Geometry check sheet. Reference: the model listing, model coordinates, mm. Round coordinates to 2 decimals unless told otherwise and drop trailing zeros. Write each loop counter-clockwise with the first axis right and the second up, starting at its lowest first coordinate (ties: lowest second). Pieces come first, ordered by that corner, then holes. Notation, with made-up numbers: M 14,87.5 L 20,87.5 A18 cw 20,101.5 Z; hole C 14.5,61 d9. An arc over 180 degrees is marked long. One line per item, written item: value. Start each with the question number.
1. Depth check by flat-ended pin: P1, Ø5, axis at y = -12, z = 37.5, coming from the +X side; P2, Ø6, axis at y = -19.5, z = 45.5, coming from the +X side; P3, Ø10, axis at y = -15, z = 27, coming from the -X side. Enter the tip coordinate at first touch or a pass-through.
2. Release check for a two-part mould opening along Z. For faces 1 (the flat face through (207, -23, 68)), 2 (the cylindrical face through (282.717, -11.339, -26.81)), 3 (the cylindrical face through (279.922, -11.099, -25.652)) record: pulls with the +Z half, pulls with the -Z half, needs draft (parallel to the pull), parting line crosses it, or undercut.
3. Section check A-A (z = 0). Record the boundary of the cut face in (x, y), and give its area (3 significant figures).
4. Scan lines: probe 1 along X at (y, z) = (-8.5, 18.5); probe 2 along Z at (x, y) = (224.5, -13.5); probe 3 along Z at (x, y) = (197.5, -2.5). Record each from-to range of solid material in increasing order. Write a range as [from, to].
5. Section check B-B (y = -13.5). Record the boundary of the cut face in (x, z) (3 decimals).
from build123d import *

# Parameters (mm, degrees)
F0_R     = 70
F0_R_2   = 66.975
F1_DEPTH = 23
F2_SIZE  = 1
F3_SIZE  = 0.5


with BuildPart() as f1:
    # F0 (on Front) → F1 (new body)
    with BuildSketch(Plane.XZ):
        with Locations((218.054354, 0)):
            Circle(F0_R)
        with Locations((218.054354, 0)):
            Circle(F0_R_2, mode=Mode.SUBTRACT)
    extrude(amount=F1_DEPTH)

    # F2
    f2_edges = [f1.edges().sort_by_distance(p)[0] for p in [
        (151.079354, -23, 0),
    ]]
    chamfer(f2_edges, length=F2_SIZE)

    # F3
    f3_edges = [f1.edges().sort_by_distance(p)[0] for p in [
        (151.079354, 0, 0),
    ]]
    chamfer(f3_edges, length=F3_SIZE)


solid = f1.part
Result sheet:
1. P1: stops at x = 278.68
1. P2: stops at x = 273.68
1. P3: stops at x = 151.6
2. face 1: needs draft
2. face 2: parting line crosses it
2. face 3: undercut
3. outline: M 148.05,-23 L 150.08,-23 L 151.08,-22 L 151.08,-0.5 L 150.58,0 L 148.05,0 Z; M 285.03,-22 L 286.03,-23 L 288.05,-23 L 288.05,0 L 285.53,0 L 285.03,-0.5 Z
3. area: 138 mm2
4. probe 1: x = [150.54, 153.69], [282.42, 285.57]
4. probe 2: z = [-69.7, -66.66], [66.66, 69.7]
4. probe 3: z = [-66.91, -63.74], [63.74, 66.91]
5. outline: C 218.054,0 d140; hole C 218.054,0 d133.95
